Input: dimensioned drawing with shaded views. Units: mm. Origin: part minimum x, y, z. A direction names the side the tool comes from. Give positions to 0.01 mm unless a question says otherwise; leave off trailing zeros. Write each loop counter-clockwise with the first axis right and the second up, starting at its lowest first coordinate (ties: lowest second). Pieces come first, ordered by that corner, then holes. Notation, with made-up numbers: (-9.75, -10) - (-4.75, -10) arc R29 cw to (-4.75, 27) - close; hole circle Ø10 at (85, -15.75). An arc over 180 degrees is marked (long way). Answer as CSV lines item,"result".
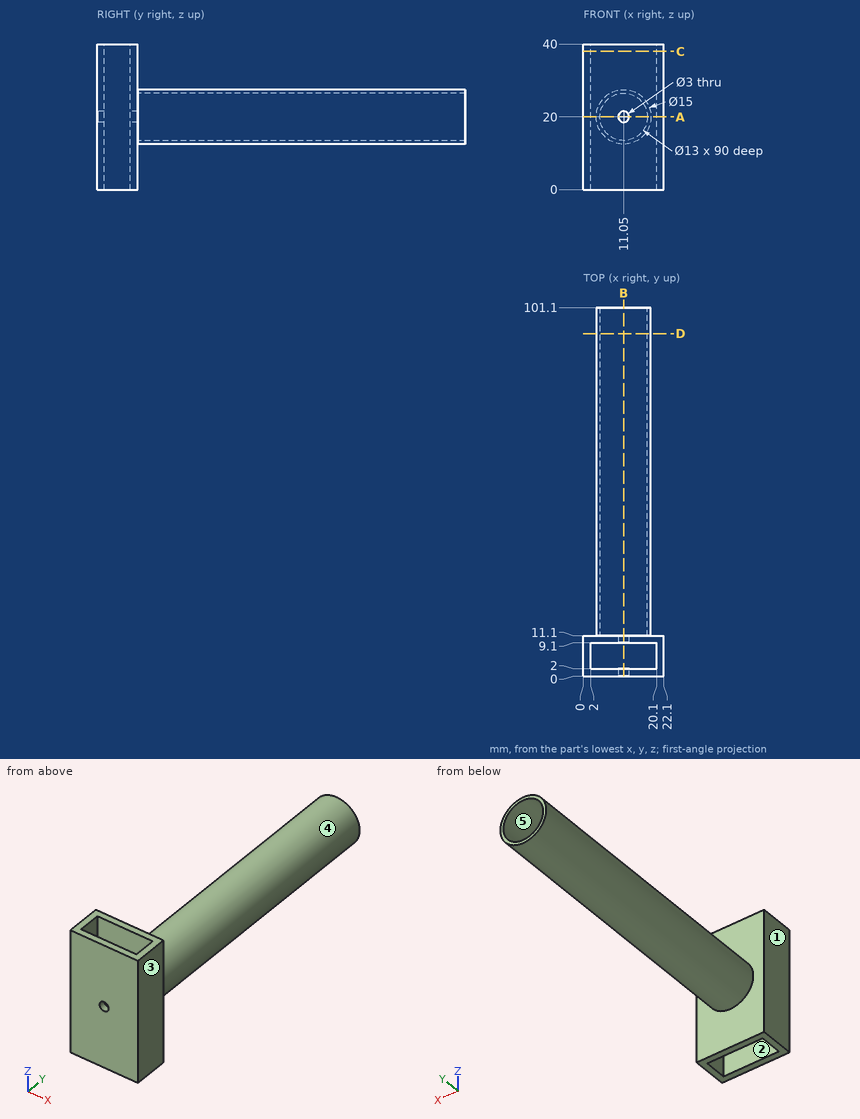
Item 1: Ray query, line 1 (Y direction, x = 18.25, z = 20.5); line 2 (Z direction, x = 11.05, y = 9.55); line 3 (X direction, y = 75, z = 20). Return the intervals inside material, ascending. Write a range as from..to.
The answers:
line 1,"0..2, 9.1..101.1"
line 2,"0..18.5, 21.5..40"
line 3,"3.55..4.55, 17.55..18.55"
Item 2: Cut plane D-D on y = 94. Return the cut outline in (x, z), plus the area to 3 significant figures.
The answers:
outline,"circle Ø15 at (11.05, 20); hole circle Ø13 at (11.05, 20)"
area,"44.0 mm²"
Item 3: Cut plane A-A on z = 20. Return the cut outline in (x, y), plus the area to 3 significant figures.
The answers:
outline,"(0, 0) - (9.55, 0) - (9.55, 2) - (2, 2) - (2, 9.1) - (9.55, 9.1) - (9.55, 11.1) - (4.55, 11.1) - (4.55, 101.1) - (3.55, 101.1) - (3.55, 11.1) - (0, 11.1) - close; (12.55, 0) - (22.1, 0) - (22.1, 11.1) - (18.55, 11.1) - (18.55, 101.1) - (17.55, 101.1) - (17.55, 11.1) - (12.55, 11.1) - (12.55, 9.1) - (20.1, 9.1) - (20.1, 2) - (12.55, 2) - close"
area,"285 mm²"
Item 4: Mould query, pull axis Z, two halves, no side actions, for the marked faces 3, 4 and 5. Classes: +Z half, -Z half, draft (parallel to the pull), parting line (faces both ways), or undercut.
The answers:
face 3,"draft"
face 4,"parting line"
face 5,"undercut"
Item 5: Reachability of the marked faces 1 and 2 from +Z, -Z, +X, -X, +Y, -Y: full face, straight path, thin tool, end or side. Return the list, or none.
The answers:
face 1,"+Z, -Z, -X, +Y, -Y"
face 2,"+Z, -Z"
Item 6: Cut plane B-B on x = 11.05. Return the cut outline in (y, z), plus the area to 3 significant figures.
The answers:
outline,"(0, 0) - (2, 0) - (2, 18.5) - (0, 18.5) - close; (0, 21.5) - (2, 21.5) - (2, 40) - (0, 40) - close; (9.1, 0) - (11.1, 0) - (11.1, 12.5) - (101.1, 12.5) - (101.1, 13.5) - (11.1, 13.5) - (11.1, 18.5) - (9.1, 18.5) - close; (9.1, 21.5) - (11.1, 21.5) - (11.1, 26.5) - (101.1, 26.5) - (101.1, 27.5) - (11.1, 27.5) - (11.1, 40) - (9.1, 40) - close"
area,"328 mm²"
Item 7: Cut plane C-C on z = 38. Return the cut outline in (x, y).
The answers:
outline,"(0, 0) - (22.1, 0) - (22.1, 11.1) - (0, 11.1) - close; hole (2, 2) - (20.1, 2) - (20.1, 9.1) - (2, 9.1) - close"
Item 8: Contact query for flat-ended pins moving along their axis: pin 1 (6 mm diameter, centred on y = 46, z = 26, fed in from +X); pin 2 (8 mm diameter, centred on x = 11.05, z = 20, fed in from +Y); pin 3 (3 mm diameter, centred on y = 30, z = 18.5, fed in from -X). Output: stop coordinate, or through.
The answers:
pin 1,"x = 17.92"
pin 2,"y = 11.1"
pin 3,"x = 3.55"
